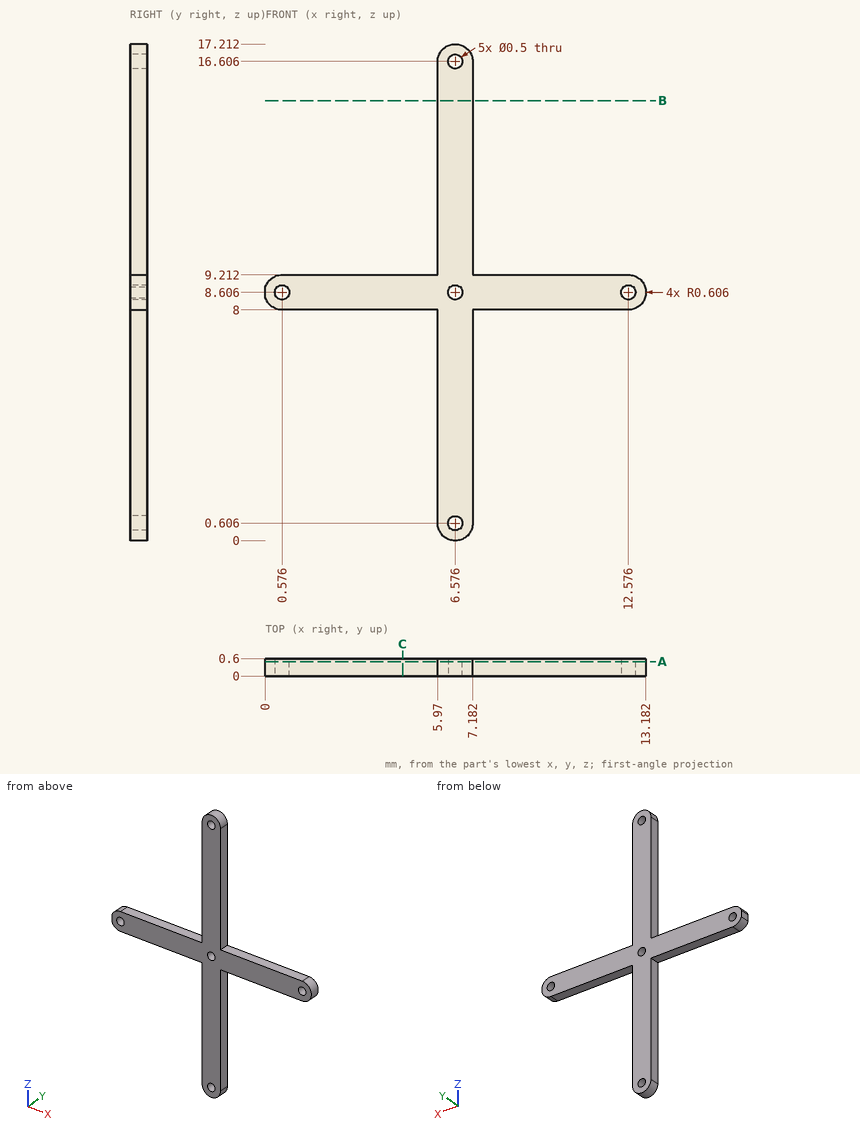
Part print with two shaded views. Sizes in mm from the minimum x, y, z corner. Coordinates: 2 decimals unless noted, no trailing zeros. Write each loop counter-clockwise with the first axis right and the second up, starting at its lowest first coordinate (ties: lowest second). Pieces come first, ordered by that corner, then holes. Notation, with made-up numbers: (8.25, -20) - (50.25, -20) arc R17 ccw to (50.25, 4) - close; hole circle Ø7 at (12, 41.5). An arc over 180 degrees is marked (long way). Put each result on its own line as item: value.
1. Band-saw the part on A-A (y = 0.5). Give the number of separate pieces and of enclosed holes in the cut face.
Final values:
separate pieces: 1
enclosed holes: 5
2. Probe line 1 along Z through (x, y) = (5.25, 0.45); line 2 along X through (y, z) = (0.1, 13); line 3 along Z through (x, y) = (12.5, 0.45) (1 decimal). List the from-to ranges inside material, lowest first. Write a range as [from, to].
Final values:
line 1: z = [8, 9.21]
line 2: x = [5.97, 7.18]
line 3: z = [8, 8.4], [8.8, 9.2]
3. Band-saw the part on C-C (x = 4.75). Write the cut outline in (y, z).
Final values:
outline: (0, 8) - (0.6, 8) - (0.6, 9.21) - (0, 9.21) - close
4. Band-saw the part on B-B (z = 15.25). Write the cut outline in (x, y).
Final values:
outline: (5.97, 0) - (7.18, 0) - (7.18, 0.6) - (5.97, 0.6) - close
